Design review of the part built by this model. Coordinates are the model's own, in mm. Face numbers are marked on the shaded views. A direction names the side the tool comes from. Coordinates: 2 decimals unless noted, no trailing zeros. Loops run counter-clockwise (first coordinate to the right, second up) from the corner with the lowest first, then second, coordinate; pieces in that order, holes last. Notation, with made-up numbers: (18.25, -12) -> (24.25, -12) arc R31 ccw to (24.25, 27) -> close; hole circle Ø7 at (45, 40.5). An arc over 180 degrees is marked (long way). Answer in a Markdown table with one row per item.
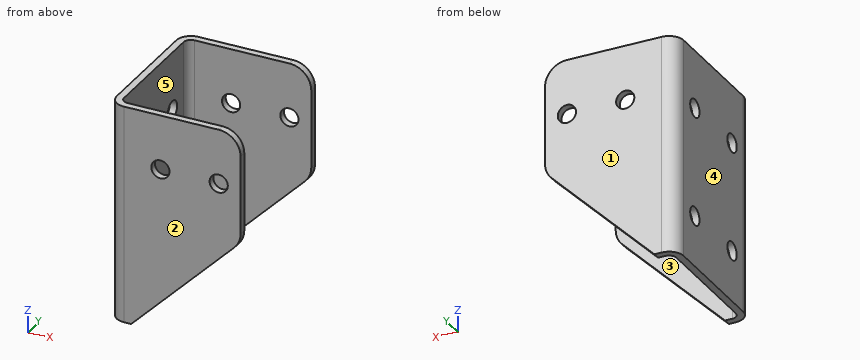
```python
from build123d import *

# Parameters (mm, degrees)
F1_DEPTH = 150
F2_R     = 6.25
F3_DEPTH = 100.001
F4_R     = 6.25
F5_DEPTH = 90.001
F6_R     = 15


with BuildPart() as f1:
    # F0 (on Top) → F1 (new body)
    with BuildSketch(Plane.XY):
        with BuildLine():
            ThreePointArc((50, 40), (47.0710678119, 47.0710678119), (40, 50))
            Line((40, 50), (-40, 50))
            ThreePointArc((-40, 50), (-47.0710678119, 47.0710678119), (-50, 40))
            Line((-50, 40), (-50, -40))
            ThreePointArc((-50, -40), (-47.0710678119, -47.0710678119), (-40, -50))
            Line((-40, -50), (40, -50))
            ThreePointArc((40, -50), (47.0710678119, -47.0710678119), (50, -40))
            Line((50, -40), (50, 40))
        make_face()
        with BuildLine():
            ThreePointArc((40, 45.0000017881), (43.5355351703, 43.5355351703), (45.0000017881, 40))
            Line((45.0000017881, 40), (45.0000017881, -40))
            ThreePointArc((45.0000017881, -40), (43.5355351703, -43.5355351703), (40, -45.0000017881))
            Line((40, -45.0000017881), (-40, -45.0000017881))
            ThreePointArc((-40, -45.0000017881), (-43.5355351703, -43.5355351703), (-45.0000017881, -40))
            Line((-45.0000017881, -40), (-45.0000017881, 40))
            ThreePointArc((-45.0000017881, 40), (-43.5355351703, 43.5355351703), (-40, 45.0000017881))
            Line((-40, 45.0000017881), (40, 45.0000017881))
        make_face(mode=Mode.SUBTRACT)
    extrude(amount=F1_DEPTH)

    # F2 (on face) → F3 (cut, through all)
    with BuildSketch(Plane.XZ.offset(50)):
        Polygon((50, 150), (40, 150), (40, 75), (-35, 0), (50, 0), align=None)
        with Locations((-15, 112.5)):
            Circle(F2_R)
        with Locations((25, 112.5)):
            Circle(F2_R)
    extrude(amount=-F3_DEPTH, mode=Mode.SUBTRACT)

    # F4 (on face) → F5 (cut, through all)
    with BuildSketch(Plane(origin=(-50, 0, 0), x_dir=(0, -1, 0), z_dir=(-1, 0, 0))):
        with Locations((-25, 110)):
            Circle(F4_R)
        with Locations((-25, 35)):
            Circle(F4_R)
        with Locations((25, 35)):
            Circle(F4_R)
        with Locations((25, 110)):
            Circle(F4_R)
    extrude(amount=-F5_DEPTH, mode=Mode.SUBTRACT)

    # F6
    f6_edges = [f1.edges().sort_by_distance(p)[0] for p in [
        (40, -47.500001, 75),
        (40, -47.500001, 150),
        (40, 47.500001, 150),
        (40, 47.500001, 75),
    ]]
    fillet(f6_edges, radius=F6_R)


solid = f1.part
```
(1) Tool access review of the marked faces 4 and 5: name each direction out of +Z, -Z, +X, -X, +Y, -Y from which nothing blocks a thin tool from reaching the whole face with its end or side.
Evaluation:
| item | result |
|---|---|
| face 4 | +Z, -Z, -X, +Y, -Y |
| face 5 | +Z, -Z, +X |
(2) To check wall thickness, follow probe 1 along Y at (x, z) = (25, 124); probe 2 along Y at (x, z) = (-46, 105.5); probe 3 along X at (y, z) = (-3.5, 23). State the ranges of each line that lie inside material, in increasing order.
Evaluation:
| item | result |
|---|---|
| probe 1 | y = -50 to -45, 45 to 50 |
| probe 2 | y = -48 to -29.34, -20.66 to 20.66, 29.34 to 48 |
| probe 3 | x = -50 to -45 |
(3) Take a section at A-A on y = 25. Give the boundary of the cut face in (x, z).
Evaluation:
| item | result |
|---|---|
| outline | (-50, 0) -> (-45, 0) -> (-45, 28.75) -> (-50, 28.75) -> close; (-50, 41.25) -> (-45, 41.25) -> (-45, 103.75) -> (-50, 103.75) -> close; (-50, 116.25) -> (-45, 116.25) -> (-45, 150) -> (-50, 150) -> close |
(4) Draft analysis for pull direction Y (two halves, no side actions). For the marked faces 1, 2 and 3, state which applies: pulls with the +Y half, pulls with the -Y half, needs draft (parallel to the pull), parting line crosses it, or undercut.
Evaluation:
| item | result |
|---|---|
| face 1 | pulls with the +Y half |
| face 2 | pulls with the -Y half |
| face 3 | undercut |
(5) Take a section at B-B on z = 35. Give the boundary of the cut face in (x, y).
Evaluation:
| item | result |
|---|---|
| outline | (-50, -40) arc R10 ccw to (-40, -50) -> (0, -50) -> (0, -45) -> (-40, -45) arc R5 cw to (-45, -40) -> (-45, -31.25) -> (-50, -31.25) -> close; (-50, -18.75) -> (-45, -18.75) -> (-45, 18.75) -> (-50, 18.75) -> close; (-50, 31.25) -> (-45, 31.25) -> (-45, 40) arc R5 cw to (-40, 45) -> (0, 45) -> (0, 50) -> (-40, 50) arc R10 ccw to (-50, 40) -> close |
(6) Take a section at D-D on x = -25.5. Give the boundary of the cut face in (y, z).
Evaluation:
| item | result |
|---|---|
| outline | (-50, 9.5) -> (-45, 9.5) -> (-45, 150) -> (-50, 150) -> close; (45, 9.5) -> (50, 9.5) -> (50, 150) -> (45, 150) -> close |
(7) Take a section at C-C on x = -15. Give the boundary of the cut face in (y, z), and give its area (4 significant figures).
Evaluation:
| item | result |
|---|---|
| outline | (-50, 20) -> (-45, 20) -> (-45, 106.25) -> (-50, 106.25) -> close; (-50, 118.75) -> (-45, 118.75) -> (-45, 150) -> (-50, 150) -> close; (45, 20) -> (50, 20) -> (50, 106.25) -> (45, 106.25) -> close; (45, 118.75) -> (50, 118.75) -> (50, 150) -> (45, 150) -> close |
| area | 1,175 mm² |
(8) For pin 1 (4 mm diameter, centred on y = -20.5, z = 122.5, fed in from +X); pin 2 (10 mm diameter, centred on x = 25, z = 112.5, fed in from -Y), all flat-tipped, find the tip position at first contact; note any pin that passes through.
Evaluation:
| item | result |
|---|---|
| pin 1 | stops at x = -45 |
| pin 2 | passes through |
